Check sheet for the modelled part. Datum: model origin and axes. Units: mm. Face numbers are marked on the shaded views. Round coordinates to 2 decimals unless told otherwise and drop trailing zeros. Write each loop counter-clockwise with the first axis right and the second up, starting at its lowest first coordinate (ties: lowest second). Pieces come first, ordered by that corner, then holes.
Item 1: Section check A-A, the plane x = 0. Record the cut outline in (y, z).
Item 2: Section check B-B, the plane y = 12.5. Record the cut outline in (x, z).
Item 3: Depth check by flat-ended pin: pin 1 (1 mm diameter, centred on x = -17, z = 15, fed in from -Y); pin 2 (1 mm diameter, centred on y = 19, z = 4.5, fed in from -X); pin 3 (5 mm diameter, centred on x = -22, z = 26.5, fed in from -Y). Enter the tip coordinate at first touch or a pass-through.
Item 4: Release check for a two-part mould opening along Y. For the marked faces 1, 2, 3 and 4 record: pulls with the +Y half, pulls with the -Y half, needs draft (parallel to the pull), parting line crosses it, or undercut.
Item 5: Material ranges on line 1 along Y through (x, z) = (0, 14); line 2 along X through (y, z) = (2.5, 24); line 3 along X through (y, z) = (-1, 14.5), recorded low to high.
Item 6: Section check D-D, the plane y = 2. Record the cut outline in (x, z), plus the area to 3 significant figures.
Item 7: Section check C-C, the plane x = 12. Record the cut outline in (y, z).
from build123d import *

# Parameters (mm, degrees)
CROQUIS1_R              = 30
CROQUIS1_R_2            = 28
SALIENTE_EXTRUIR1_DEPTH = 23
CROQUIS2_R              = 1.15
SALIENTE_EXTRUIR2_DEPTH = 2
CROQUIS4_R              = 30
CROQUIS4_R_2            = 24.5
SALIENTE_EXTRUIR3_DEPTH = 2
CROQUIS5_R              = 30
CROQUIS5_R_2            = 26.2
SALIENTE_EXTRUIR4_DEPTH = 7


with BuildPart() as part:
    # Croquis1 → Saliente-Extruir1 (new body)
    with BuildSketch(Plane.XY):
        Circle(CROQUIS1_R)
        Circle(CROQUIS1_R_2, mode=Mode.SUBTRACT)
    extrude(amount=SALIENTE_EXTRUIR1_DEPTH)

    # Croquis2 → Saliente-Extruir2 (add)
    # profile 1 of 5: a face of its own
    with BuildSketch(Plane.XY):
        with BuildLine():
            Line((-3, 25), (-3.336066177, 27.800551478))
            ThreePointArc((-3.336066177, 27.800551478), (0, 28), (3.336066177, 27.800551478))
            Line((3.336066177, 27.800551478), (3, 25))
            ThreePointArc((3, 25), (0, 22), (-3, 25))
        make_face()
        with Locations((0, 25)):
            Circle(CROQUIS2_R, mode=Mode.SUBTRACT)
    # profile 2 of 5: a face of its own
    with BuildSketch(Plane.XY):
        with BuildLine():
            Line((20.150635095, 15.098076211), (22.40795073, 16.789393797))
            ThreePointArc((22.40795073, 16.789393797), (24.248711306, 14), (25.744016908, 11.011157681))
            Line((25.744016908, 11.011157681), (23.150635095, 9.901923789))
            ThreePointArc((23.150635095, 9.901923789), (19.052558883, 11), (20.150635095, 15.098076211))
        make_face()
        with Locations((21.650635095, 12.5)):
            Circle(CROQUIS2_R, mode=Mode.SUBTRACT)
    # profile 3 of 5: a face of its own
    with BuildSketch(Plane.XY):
        with BuildLine():
            Line((23.150635095, -9.901923789), (25.744016908, -11.011157681))
            ThreePointArc((25.744016908, -11.011157681), (24.248711306, -14), (22.40795073, -16.789393797))
            Line((22.40795073, -16.789393797), (20.150635095, -15.098076211))
            ThreePointArc((20.150635095, -15.098076211), (19.052558883, -11), (23.150635095, -9.901923789))
        make_face()
        with Locations((21.650635095, -12.5)):
            Circle(CROQUIS2_R, mode=Mode.SUBTRACT)
    # profile 4 of 5: a face of its own
    with BuildSketch(Plane.XY):
        with BuildLine():
            Line((-20.150635095, -15.098076211), (-22.40795073, -16.789393797))
            ThreePointArc((-22.40795073, -16.789393797), (-24.248711306, -14), (-25.744016908, -11.011157681))
            Line((-25.744016908, -11.011157681), (-23.150635095, -9.901923789))
            ThreePointArc((-23.150635095, -9.901923789), (-19.052558883, -11), (-20.150635095, -15.098076211))
        make_face()
        with Locations((-21.650635095, -12.5)):
            Circle(CROQUIS2_R, mode=Mode.SUBTRACT)
    # profile 5 of 5: a face of its own
    with BuildSketch(Plane.XY):
        with BuildLine():
            Line((-23.150635095, 9.901923789), (-25.744016908, 11.011157681))
            ThreePointArc((-25.744016908, 11.011157681), (-24.248711306, 14), (-22.40795073, 16.789393797))
            Line((-22.40795073, 16.789393797), (-20.150635095, 15.098076211))
            ThreePointArc((-20.150635095, 15.098076211), (-19.052558883, 11), (-23.150635095, 9.901923789))
        make_face()
        with Locations((-21.650635095, 12.5)):
            Circle(CROQUIS2_R, mode=Mode.SUBTRACT)
    extrude(amount=SALIENTE_EXTRUIR2_DEPTH)

    # Croquis4 → Saliente-Extruir3 (add)
    with BuildSketch(Plane.XY.offset(23)):
        Circle(CROQUIS4_R)
        Circle(CROQUIS4_R_2, mode=Mode.SUBTRACT)
    extrude(amount=SALIENTE_EXTRUIR3_DEPTH)

    # Croquis5 → Saliente-Extruir4 (add)
    with BuildSketch(Plane.XY.offset(25)):
        Circle(CROQUIS5_R)
        Circle(CROQUIS5_R_2, mode=Mode.SUBTRACT)
    extrude(amount=SALIENTE_EXTRUIR4_DEPTH)


solid = part.part
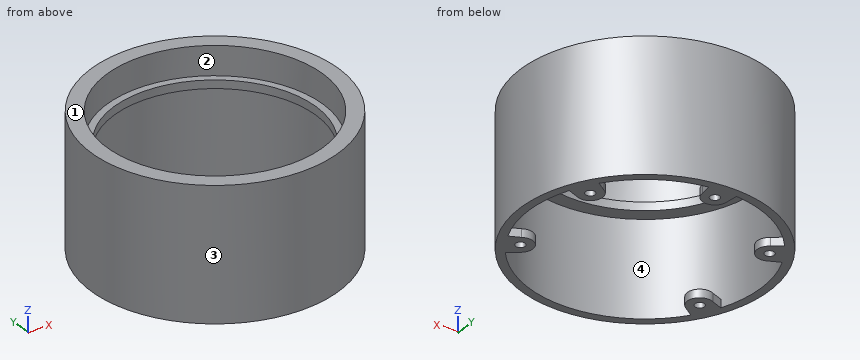
Values found:
1. outline: (-30, 0) - (-28, 0) - (-28, 23) - (-24.5, 23) - (-24.5, 25) - (-26.2, 25) - (-26.2, 32) - (-30, 32) - close; (22, 0) - (23.85, 0) - (23.85, 2) - (22, 2) - close; (24.5, 23) - (28, 23) - (28, 2) - (26.15, 2) - (26.15, 0) - (30, 0) - (30, 32) - (26.2, 32) - (26.2, 25) - (24.5, 25) - close
2. outline: (-27.27, 0) - (-22.8, 0) - (-22.8, 2) - (-25.05, 2) - (-25.05, 23) - (-21.07, 23) - (-21.07, 25) - (-23.03, 25) - (-23.03, 32) - (-27.27, 32) - close; (-20.5, 0) - (-18.65, 0) - (-18.65, 2) - (-20.5, 2) - close; (18.65, 0) - (20.5, 0) - (20.5, 2) - (18.65, 2) - close; (21.07, 23) - (25.05, 23) - (25.05, 2) - (22.8, 2) - (22.8, 0) - (27.27, 0) - (27.27, 32) - (23.03, 32) - (23.03, 25) - (21.07, 25) - close
3. pin 1: stops at y = -25.05
3. pin 2: stops at x = -23.62
3. pin 3: stops at y = -22.8
4. face 1: needs draft
4. face 2: undercut
4. face 3: parting line crosses it
4. face 4: undercut
5. line 1: y = -30 to -28, 28 to 30
5. line 2: x = -29.9 to -24.37, 24.37 to 29.9
5. line 3: x = -29.98 to -27.98, 27.98 to 29.98
6. outline: (-29.93, 0) - (-27.93, 0) - (-27.93, 23) - (-24.42, 23) - (-24.42, 25) - (-26.12, 25) - (-26.12, 32) - (-29.93, 32) - close; (24.42, 23) - (27.93, 23) - (27.93, 0) - (29.93, 0) - (29.93, 32) - (26.12, 32) - (26.12, 25) - (24.42, 25) - close
6. area: 168 mm2
7. outline: (-27.5, 0) - (-25.3, 0) - (-25.3, 23) - (-21.36, 23) - (-21.36, 25) - (-23.29, 25) - (-23.29, 32) - (-27.5, 32) - close; (21.36, 23) - (25.3, 23) - (25.3, 0) - (27.5, 0) - (27.5, 32) - (23.29, 32) - (23.29, 25) - (21.36, 25) - close
